from build123d import *

# Parameters (mm, degrees)
Y_KSEKLIK_EKSTR_ZYON1_DEPTH = 4
KES_EKSTR_ZYON1_START       = -4
KES_EKSTR_ZYON1_DEPTH       = 4
IZIM3_R                     = 5
KES_EKSTR_ZYON2_DEPTH       = 4
KES_EKSTR_ZYON3_DEPTH       = 4
IZIM10_R                    = 7.25
IZIM10_R_2                  = 5
KES_EKSTR_ZYON4_DEPTH       = 3.5
IZIM11_R                    = 5
Y_KSEKLIK_EKSTR_ZYON3_DEPTH = 2
PAH2_SIZE                   = 1


with BuildPart() as part:
    # Çizim1 → Yükseklik-Ekstrüzyon1 (new body)
    with BuildSketch(Plane.XY):
        with BuildLine():
            Line((-35.653037037, 15), (24.346962963, 15))
            ThreePointArc((24.346962963, 15), (39.346962963, 0), (24.346962963, -15))
            Line((24.346962963, -15), (-35.653037037, -15))
            ThreePointArc((-35.653037037, -15), (-50.653037037, 0), (-35.653037037, 15))
        make_face()
    extrude(amount=Y_KSEKLIK_EKSTR_ZYON1_DEPTH)

    # Çizim2 → Kes-Ekstrüzyon1 (cut)
    with BuildSketch(Plane.XY.offset(4).offset(KES_EKSTR_ZYON1_START)):
        Polygon((-11.560212186, 15), (-35.653037037, 15), (-33.243754552, 4.590717515), (-10.375990279, 9.883580305), align=None)
        Polygon((-33.243754552, -4.590717515), (-35.653037037, -15), (-11.560212186, -15), (-10.375990279, -9.883580305), align=None)
        with BuildLine():
            Line((-10.375990279, 9.883580305), (-9.150929701, 4.590717515))
            Line((-9.150929701, 4.590717515), (30.369414779, 13.737906468))
            ThreePointArc((30.369414779, 13.737906468), (27.42360098, 14.681086421), (24.346962963, 15))
            Line((24.346962963, 15), (11.729453249, 15))
            Line((11.729453249, 15), (-10.375990279, 9.883580305))
        make_face()
        with BuildLine():
            Line((-9.150929701, -4.590717515), (-10.375990279, -9.883580305))
            Line((-10.375990279, -9.883580305), (11.729453249, -15))
            Line((11.729453249, -15), (24.346962963, -15))
            ThreePointArc((24.346962963, -15), (27.42360098, -14.681086421), (30.369414779, -13.737906468))
            Line((30.369414779, -13.737906468), (-9.150929701, -4.590717515))
        make_face()
    extrude(amount=KES_EKSTR_ZYON1_DEPTH, mode=Mode.SUBTRACT)


with BuildPart() as kes_ekstr_zyon1_piece_1:
    # of the separate pieces the step leaves, piece 1, a body of its own (kes_ekstr_zyon1_pieces)
    add(part.part.solids().sort_by_distance((-35.653037037, -15, 0))[0])

    # Çizim3 → Kes-Ekstrüzyon2 (cut)
    with BuildSketch(Plane.XY.offset(4)):
        with Locations((24.346962963, 0)):
            Circle(IZIM3_R)
    extrude(amount=-KES_EKSTR_ZYON2_DEPTH, mode=Mode.SUBTRACT)

    # Çizim10 → Kes-Ekstrüzyon4 (cut)
    # profile 1 of 2: a face of its own
    with BuildSketch(Plane.XY.offset(4)):
        with BuildLine():
            ThreePointArc((22.99921211, -7.123627421), (17.102780918, 0.290390243), (23.573735665, 7.20864894))
            Line((23.573735665, 7.20864894), (5.173034472, 5.234919246))
            ThreePointArc((5.173034472, 5.234919246), (0.709580704, 0.698667438), (5.245832511, -3.76478633))
            Line((5.245832511, -3.76478633), (22.99921211, -7.123627421))
        make_face()
    # profile 2 of 2: a face of its own
    with BuildSketch(Plane.XY.offset(4)):
        with Locations((24.346962963, 0)):
            Circle(IZIM10_R)
        with Locations((24.346962963, 0)):
            Circle(IZIM10_R_2, mode=Mode.SUBTRACT)
    extrude(amount=-KES_EKSTR_ZYON4_DEPTH, mode=Mode.SUBTRACT)

    # Çizim11 → Yükseklik-Ekstrüzyon3 (add)
    with BuildSketch(Plane(origin=(0, 0, 0), x_dir=(-1, 0, 0), z_dir=(0, 0, -1))):
        with BuildLine():
            Line((33.243754552, -4.590717515), (35.653037037, -15))
            ThreePointArc((35.653037037, -15), (50.653037037, 0), (35.653037037, 15))
            Line((35.653037037, 15), (33.243754552, 4.590717515))
            Line((33.243754552, 4.590717515), (10.375990279, 9.883580305))
            Line((10.375990279, 9.883580305), (9.150929701, 4.590717515))
            Line((9.150929701, 4.590717515), (-30.369414779, 13.737906468))
            ThreePointArc((-30.369414779, 13.737906468), (-39.346962963, 0), (-30.369414779, -13.737906468))
            Line((-30.369414779, -13.737906468), (9.150929701, -4.590717515))
            Line((9.150929701, -4.590717515), (10.375990279, -9.883580305))
            Line((10.375990279, -9.883580305), (33.243754552, -4.590717515))
        make_face()
        with Locations(Location((-24.346962963, 0, 0), (0, 0, 180))):
            Circle(IZIM11_R, mode=Mode.SUBTRACT)
    extrude(amount=Y_KSEKLIK_EKSTR_ZYON3_DEPTH)

    # Pah2
    pah2_edges = [kes_ekstr_zyon1_piece_1.edges().sort_by_distance(p)[0] for p in [
        (19.346962963, 0, 0.5),
    ]]
    chamfer(pah2_edges, length=PAH2_SIZE)


with BuildPart() as kes_ekstr_zyon1_piece_2:
    # of the separate pieces the step leaves, piece 2, a body of its own (kes_ekstr_zyon1_pieces)
    add(part.part.solids().sort_by_distance((-11.560212186, 15, 0))[0])


with BuildPart() as kes_ekstr_zyon1_piece_3:
    # of the separate pieces the step leaves, piece 3, a body of its own (kes_ekstr_zyon1_pieces)
    add(part.part.solids().sort_by_distance((11.729453249, -15, 0))[0])


with BuildPart() as kes_ekstr_zyon3_tool:
    # Çizim5 → Kes-Ekstrüzyon3 (new body)
    with BuildSketch(Plane.XY.offset(4)):
        Polygon((-10.375990279, -9.883580305), (-11.560212186, -15), (11.729453249, -15), align=None)
        Polygon((-11.560212186, 15), (-10.375990279, 9.883580305), (11.729453249, 15), align=None)
    extrude(amount=-KES_EKSTR_ZYON3_DEPTH)


with BuildPart() as kes_ekstr_zyon1_piece_2_1:
    add(kes_ekstr_zyon1_piece_2.part)

    # Kes-Ekstrüzyon3: cut by kes_ekstr_zyon3_tool
    add(kes_ekstr_zyon3_tool.part, mode=Mode.SUBTRACT)


with BuildPart() as kes_ekstr_zyon1_piece_3_1:
    add(kes_ekstr_zyon1_piece_3.part)

    # Kes-Ekstrüzyon3: cut by kes_ekstr_zyon3_tool
    add(kes_ekstr_zyon3_tool.part, mode=Mode.SUBTRACT)


solid = kes_ekstr_zyon1_piece_1.part
Geometry: final body of the model. Coordinates: model frame, mm. A direction names the side the tool comes from. Round coordinates to 2 decimals unless told otherwise and drop trailing zeros. Loops run counter-clockwise (first coordinate to the right, second up) from the corner with the lowest first, then second, coordinate; pieces in that order, holes last. Notation, with made-up numbers: (48.25, -4.5) -> (82.25, -4.5) arc R18 cw to (82.25, 27.5) -> close; hole circle Ø11 at (-24, 67.5). An arc over 180 degrees is marked (long way). One line per question, with ' | ' between items. Start each with the question number.
1. Section C-C on x = 3. Output: boundary loops of the cut face in (y, z), and give its area (3 significant figures).
2. Line query: line 1 along X through (y, z) = (0, -1.15); line 2 along Y through (x, z) = (-36, 2); line 3 along Y through (x, z) = (11, 1.55). Output: solid intervals per line, ascending. Write a range as [from, to].
3. Set-up query: faces 1 (the face through (14, -5.42, 2.27)), 2 (the face through (-5, 0, 4)), 3 (the face through (29.116, -1.502, -1.24)), 4 (the face through (-21.97, 7.2, 1.04)), 5 (the face through (-9.755, -7.2, 1.042)). Return all of +Z, -Z, +X, -X, +Y, -Y with unobstructed straight access to the full face (end or side cutting, diameter ignored); none if empty.
4. Mould query, pull axis X, two halves, no side actions, for faces 6 (the face through (-9.77, 7.27, 1.04)), 7 (the face through (0.71, 0.8, 2.27)), 8 (the face through (-50.65, -0.33, 1.04)), 9 (the face through (-5, 0, -2)). Classes: pulls with the +X half, pulls with the -X half, needs draft (parallel to the pull), parting line crosses it, or undercut.
5. Section A-A on z = 3.2. Output: boundary loops of the cut face in (x, y).
6. Section D-D on y = -12.75. Output: boundary loops of the cut face in (x, z), and give its area (3 significant figures).
7. Section B-B on y = 0. Output: boundary loops of the cut face in (x, z).
8. Contact query for flat-ended pins moving along their axis: pin 1 (7 mm diameter, centred on x = 22.5, y = 2.5, fed in from +Z); pin 2 (1.5 mm diameter, centred on y = -5.5, z = 2.5, fed in from +X) (3 decimals); pin 3 (3 mm diameter, centred on y = 5, z = 0.5, fed in from +X). Output: stop coordinate, or through.
Returned:
1) outline: (-7.4, -2) -> (7.4, -2) -> (7.4, 4) -> (4.66, 4) -> (4.66, 0.5) -> (-3.19, 0.5) -> (-3.19, 4) -> (-7.4, 4) -> close | area: 61.4 mm2
2) line 1: x = [-50.65, 19.35], [29.35, 39.35] | line 2: y = [-15, 15] | line 3: y = [-9.25, -4.85], [5.86, 9.25]
3) face 1: +Z | face 2: +Z, +X, -X, +Y, -Y | face 3: +Z, -Z | face 4: +Z, -Z, +Y | face 5: +Z, -Z, -Y
4) face 6: undercut | face 7: undercut | face 8: pulls with the -X half | face 9: needs draft
5) outline: (-35.65, -15) -> (-33.24, -4.59) -> (-10.38, -9.88) -> (-9.15, -4.59) -> (30.37, -13.74) arc R15 ccw to (30.37, 13.74) -> (-9.15, 4.59) -> (-10.38, 9.88) -> (-33.24, 4.59) -> (-35.65, 15) arc R15 ccw to start; hole (5.17, 5.23) arc R4.5 ccw to (5.25, -3.76) -> (23, -7.12) arc R7.25 ccw (long way) to (23.57, 7.21) -> close
6) outline: (-43.55, -2) -> (-35.13, -2) -> (-35.13, 4) -> (-43.55, 4) -> close; (26.1, -2) -> (32.25, -2) -> (32.25, 4) -> (26.1, 4) -> close | area: 87.4 mm2
7) outline: (-50.65, -2) -> (19.35, -2) -> (19.35, -0.5) -> (18.35, 0.5) -> (0.77, 0.5) -> (0.77, 4) -> (-50.65, 4) -> close; (29.35, -2) -> (39.35, -2) -> (39.35, 4) -> (31.6, 4) -> (31.6, 0.5) -> (30.35, 0.5) -> (29.35, -0.5) -> close
8) pin 1: stops at z = 0.5 | pin 2: stops at x = 38.575 | pin 3: stops at x = 38.93
